```python
from build123d import *

# Parameters (mm, degrees)
SKETCH1_W           = 35
SKETCH1_H           = 35
BOSS_EXTRUDE1_DEPTH = 27
SKETCH2_W           = 31
SKETCH2_H           = 21
CUT_EXTRUDE1_DEPTH  = 31
CUT_EXTRUDE2_DEPTH  = 37.626493144
CUT_EXTRUDE3_DEPTH  = 45.679413604
CUT_EXTRUDE4_DEPTH  = 45.679413604
SKETCH7_W           = 31
SKETCH7_H           = 3.5
CUT_EXTRUDE5_DEPTH  = 1
SKETCH8_W           = 31
SKETCH8_H           = 3.5
CUT_EXTRUDE6_DEPTH  = 1
SKETCH9_W           = 3.5
SKETCH9_H           = 31
CUT_EXTRUDE13_DEPTH = 1
SKETCH10_W          = 3.5
SKETCH10_H          = 31
CUT_EXTRUDE14_DEPTH = 1


with BuildPart() as part:
    # Sketch1 → Boss-Extrude1 (new body)
    with BuildSketch(Plane.XY):
        Rectangle(SKETCH1_W, SKETCH1_H)
    extrude(amount=BOSS_EXTRUDE1_DEPTH)

    # Sketch2 → Cut-Extrude1 (cut)
    with BuildSketch(Plane(origin=(0, 17.5, 0), x_dir=(1, 0, 0), z_dir=(0, 1, 0))):
        with Locations((2, -13.5)):
            Rectangle(SKETCH2_W, SKETCH2_H)
    extrude(amount=-CUT_EXTRUDE1_DEPTH, mode=Mode.SUBTRACT)

    # Sketch3 → Cut-Extrude2 (cut, through all)
    with BuildSketch(Plane.XY.offset(27)):
        Polygon((17.5, 17.5), (-10.5, 17.5), (-10.5, 9.5), (9.5, -10.5), (17.5, -10.5), align=None)
    extrude(amount=-CUT_EXTRUDE2_DEPTH, mode=Mode.SUBTRACT)

    # Sketch4 → Cut-Extrude3 (cut, through all)
    with BuildSketch(Plane(origin=(-13.5, 0, 0), x_dir=(0, 0, -1), z_dir=(1, 0, 0))):
        with BuildLine():
            Line((-9.5, 7), (-9.5, -3))
            ThreePointArc((-9.5, -3), (-13.5, -7), (-17.5, -3))
            Line((-17.5, -3), (-17.5, 7))
            ThreePointArc((-17.5, 7), (-13.5, 11), (-9.5, 7))
        make_face()
    extrude(amount=-CUT_EXTRUDE3_DEPTH, mode=Mode.SUBTRACT)

    # Sketch5 → Cut-Extrude4 (cut, through all)
    with BuildSketch(Plane(origin=(0, -13.5, 0), x_dir=(1, 0, 0), z_dir=(0, 1, 0))):
        with BuildLine():
            Line((-3, -9.5), (7, -9.5))
            ThreePointArc((7, -9.5), (11, -13.5), (7, -17.5))
            Line((7, -17.5), (-3, -17.5))
            ThreePointArc((-3, -17.5), (-7, -13.5), (-3, -9.5))
        make_face()
    extrude(amount=-CUT_EXTRUDE4_DEPTH, mode=Mode.SUBTRACT)

    # Sketch7 → Cut-Extrude5 (cut)
    with BuildSketch(Plane.XZ.offset(17.5)):
        with Locations((0, 22.25)):
            Rectangle(SKETCH7_W, SKETCH7_H)
    extrude(amount=-CUT_EXTRUDE5_DEPTH, mode=Mode.SUBTRACT)

    # Sketch8 → Cut-Extrude6 (cut)
    with BuildSketch(Plane.XZ.offset(17.5)):
        with Locations((0, 4.75)):
            Rectangle(SKETCH8_W, SKETCH8_H)
    extrude(amount=-CUT_EXTRUDE6_DEPTH, mode=Mode.SUBTRACT)

    # Sketch9 → Cut-Extrude13 (cut)
    with BuildSketch(Plane.ZY.offset(17.5)):
        with Locations((22.25, 0)):
            Rectangle(SKETCH9_W, SKETCH9_H)
    extrude(amount=-CUT_EXTRUDE13_DEPTH, mode=Mode.SUBTRACT)

    # Sketch10 → Cut-Extrude14 (cut)
    with BuildSketch(Plane.ZY.offset(17.5)):
        with Locations((4.75, 0)):
            Rectangle(SKETCH10_W, SKETCH10_H)
    extrude(amount=-CUT_EXTRUDE14_DEPTH, mode=Mode.SUBTRACT)


solid = part.part
```
The model under review builds one solid part; all positions refer to its coordinate system, in mm. A direction names the side the tool comes from. Round coordinates to 2 decimals unless told otherwise and drop trailing zeros. Loops run counter-clockwise (first coordinate to the right, second up) from the corner with the lowest first, then second, coordinate; pieces in that order, holes last. Notation, with made-up numbers: (32, -4.5) - (49, -4.5) arc R15 cw to (49, 0.5) - close; hole circle Ø7 at (-29, -25.75). An arc over 180 degrees is marked (long way). Write each question's results on one line, items separated by ' | '. Start each with the question number.
Q1. Insertion check: P1, Ø2, axis at x = -5.5, z = 12.5, coming from the +Y side; P2, Ø0.9, axis at y = 13, z = 26, coming from the +X side; P3, Ø1, axis at y = 9, z = 6.5, coming from the +X side; P4, Ø1.5, axis at x = 14.5, z = 1, coming from the +Y side. Each pin has a flat end and moves straight along its axis. Give the tip position at first contact, or say it passes through.
Q2. Draft analysis for pull direction Y (two halves, no side actions). For faces 5 (the flat face through (0, -16.5, 5)), 6 (the flat face through (-15, 2, 17.5)), 7 (the flat face through (13, -10.5, 26)), 8 (the flat face through (-17, 0, 24)), state which applies: pulls with the +Y half, pulls with the -Y half, needs draft (parallel to the pull), parting line crosses it, or undercut.
Q3. Wall thickness on line 1 along Z through (x, y) = (-7.5, -13); line 2 along Y through (x, z) = (-14.5, 13.5); line 3 along Z through (x, y) = (3.5, -14.5): over which ranges is each line inside the solid? List them lowest first. Write a range as [from, to].
Q4. Take a section at C-C on y = -15. Give the boundary of the cut face in (x, z), plus the area to 3 significant figures.
Q5. Take a section at A-A on z = 13.5. Give the boundary of the cut face in (x, y), plus the area to 3 significant figures.
Q6. Take a section at D-D on x = -6. Give the boundary of the cut face in (y, z), plus the area to 3 significant figures.
Q7. Tool access review of faces 1 (the flat face through (-10.5, 14, 26)), 2 (the flat face through (2, -15, 17.5)), 3 (the flat face through (0, -17, 3)), 4 (the flat face through (2, -13.5, 9)): name each direction out of +Z, -Z, +X, -X, +Y, -Y from which nothing blocks a thin tool from reaching the whole face with its end or side.
Q8. Take a section at B-B on y = 6.5. Give the boundary of the cut face in (x, z), plus the area to 3 significant figures.
Data:
1) P1: passes through | P2: stops at x = -10.5 | P3: stops at x = -13.5 | P4: stops at y = -10.5
2) face 5: pulls with the -Y half | face 6: undercut | face 7: pulls with the +Y half | face 8: undercut
3) line 1: z = [0, 3], [24, 27] | line 2: y = [-17.5, -7], [11, 17.5] | line 3: z = [0, 9.5], [17.5, 27]
4) outline: (-17.5, 0) - (17.5, 0) - (17.5, 27) - (-17.5, 27) - (-17.5, 24) - (-16.5, 24) - (-16.5, 20.5) - (-17.5, 20.5) - (-17.5, 6.5) - (-16.5, 6.5) - (-16.5, 3) - (-17.5, 3) - close; hole (-3, 9.5) - (7, 9.5) arc R4 ccw to (7, 17.5) - (-3, 17.5) arc R4 ccw to start | area: 808 mm²
5) outline: (-17.5, -17.5) - (-7, -17.5) - (-7, -13.5) - (-13.5, -13.5) - (-13.5, -7) - (-17.5, -7) - close; (-17.5, 11) - (-13.5, 11) - (-13.5, 17.5) - (-17.5, 17.5) - close; (11, -17.5) - (17.5, -17.5) - (17.5, -13.5) - (11, -13.5) - close | area: 120 mm²
6) outline: (-17.5, 0) - (5, 0) - (5, 3) - (-13.5, 3) - (-13.5, 10.85) - (-17.5, 10.85) - (-17.5, 6.5) - (-16.5, 6.5) - (-16.5, 3) - (-17.5, 3) - close; (-17.5, 16.15) - (-13.5, 16.15) - (-13.5, 24) - (5, 24) - (5, 27) - (-17.5, 27) - (-17.5, 24) - (-16.5, 24) - (-16.5, 20.5) - (-17.5, 20.5) - close | area: 191 mm²
7) face 1: +Z, -Z, +X, +Y | face 2: +Y, -Y | face 3: -Y | face 4: +X, +Y
8) outline: (-17.5, 0) - (-7.5, 0) - (-7.5, 3) - (-13.5, 3) - (-13.5, 9.5) - (-17.5, 9.5) - (-17.5, 6.5) - (-16.5, 6.5) - (-16.5, 3) - (-17.5, 3) - close; (-17.5, 17.5) - (-13.5, 17.5) - (-13.5, 24) - (-7.5, 24) - (-7.5, 27) - (-17.5, 27) - (-17.5, 24) - (-16.5, 24) - (-16.5, 20.5) - (-17.5, 20.5) - close | area: 105 mm²
